Build history of the part. All positions in model axes, mm. Round coordinates to 2 decimals unless told otherwise and drop trailing zeros.
from build123d import *

# Parameters (mm, degrees)
BOSS_EXTRUDE1_DEPTH = 27.432
SKETCH2_R           = 5
SKETCH2_R_2         = 3.175
CUT_EXTRUDE1_DEPTH  = 317.917465392
SKETCH3_W           = 293.188888759
SKETCH3_H           = 137.971241769
CUT_EXTRUDE2_DEPTH  = 317.917465392


with BuildPart() as part:
    # Sketch1 → Boss-Extrude1 (new body)
    with BuildSketch(Plane.XY):
        with BuildLine():
            add(Edge.make_bspline(
                [(0.000560351, 0.000130087), (0.810633127, 7.359196055), (8.649092025, 17.856605174), (26.286719818, 29.975176328), (52.111128271, 42.069215275), (89.597618475, 49.290763054), (131.400792109, 47.884831915), (173.256699242, 40.041104278), (217.961060472, 29.612974894), (256.952064401, 19.528920948), (290.35983767, 8.71099439), (301.273197721, 4.382828139), (314.816918223, -0.516206742), (309.846313895, 0.000130087)],
                knots=[0, 0, 0, 0, 0.060863618, 0.113688265, 0.188608742, 0.312908923, 0.448482434, 0.557612135, 0.691544113, 0.852438279, 0.92975597, 0.976058229, 1, 1, 1, 1], degree=3))
            add(Edge.make_bspline(
                [(309.846313895, 0.000130087), (303.956832565, 1.47095521), (293.989507544, 2.093987313), (276.26402299, 4.514356704), (260.846344817, 5.427413394), (235.858814759, 7.870306192), (205.101424636, 8.838080282), (157.718638092, 9.030650149), (110.497331172, 6.181495223), (66.506197185, -0.586669107), (36.454672816, -6.098499901), (15.316603331, -6.189065841), (1.230714189, -6.924076091), (0.000560351, 0.000130087)],
                knots=[0, 0, 0, 0, 0.057787081, 0.095274891, 0.171021118, 0.205339302, 0.335319146, 0.464904334, 0.658702312, 0.785511947, 0.893517288, 0.94309214, 1, 1, 1, 1], degree=3))
        make_face()
    extrude(amount=BOSS_EXTRUDE1_DEPTH)

    # Sketch2 → Cut-Extrude1 (cut, through all)
    with BuildSketch(Plane.XY.offset(27.432)):
        with Locations((20.32, 10.16)):
            Circle(SKETCH2_R)
        with Locations((227.296313895, 19.050130087)):
            Circle(SKETCH2_R_2)
    extrude(amount=-CUT_EXTRUDE1_DEPTH, mode=Mode.SUBTRACT)

    # Sketch3 → Cut-Extrude2 (cut, through all)
    with BuildSketch(Plane.XY.offset(27.432)):
        with Locations((184.69444438, 2.732377951)):
            Rectangle(SKETCH3_W, SKETCH3_H)
    extrude(amount=-CUT_EXTRUDE2_DEPTH, mode=Mode.SUBTRACT)


solid = part.part
1) Wall check: L1, parallel to Y at x = 21, z = 21.25; L2, parallel to Y at x = 20.32, z = 14; L3, parallel to X at y = 12, z = 8.75. Give the ranges that are in metal, low to high.
Results:
L1: y = -6.19 to 5.21, 15.11 to 26.1
L2: y = -6.21 to 5.16, 15.16 to 25.66
L3: x = 4.88 to 15.67, 24.97 to 38.1
2) Pin check, flat tips, straight feed: pin 1 Ø10 at (x, z) = (5, 7) entering from +Y; pin 2 Ø8 at (x, z) = (27, 19) entering from -Y; pin 3 Ø1 at (y, z) = (-1.5, 10.5) entering from -X. Stop position of each tip, or through.
Results:
pin 1: stops at y = 17.68
pin 2: stops at y = -6.14
pin 3: stops at x = 0.24
3) Mould opens along Y. For faces 1 (the cylindrical face through (16.35, 7.12, 13.91)), 2 (the flat face through (24, 5, 0)) say: released by +Y, released by -Y, zero draft, split by the parting line, or undercut.
Results:
face 1: undercut
face 2: zero draft
